Source: CAD feature listing. Evaluate the final solid. Frame: model axes, mm. Face numbers are marked on the shaded views. A direction names the side the tool comes from. Round coordinates to 2 decimals unless told otherwise and drop trailing zeros. Loops run counter-clockwise (first coordinate to the right, second up) from the corner with the lowest first, then second, coordinate; pieces in that order, holes last.
(1) First-contact query: pin 1 Ø8.5 at (x, z) = (-58.5, 8.5) entering from +Y; pin 2 Ø6 at (y, z) = (6.5, 10) entering from -X; pin 3 Ø2 at (x, z) = (-2, 17) entering from -Y; pin 4 Ø5 at (x, z) = (78.5, 0) entering from +Y. Flat tips, straight axial feed; report the tip coordinate or a pass-through.
(2) Section D-D, the plane x = -78.5. Return the cut outline in (y, z).
(3) Section A-A, the plane y = 2.5. Count the separate pieces of the cut face and the enclosed holes in it, plus the area to 3 significant figures.
(4) Section B-B, the plane x = 5. Return the cut outline in (y, z), plus the area to 3 significant figures.
(5) Set-up query: the marked faces 1, 2, 3, 4 and 5. Return all of +Z, -Z, +X, -X, +Y, -Y with unobstructed straight access to the full face (end or side cutting, diameter ignored); none if empty.
(6) Material intervals for probe 1 along Z at (x, y) = (58.5, 1.6); probe 2 along X at (y, z) = (1.15, 8.5); probe 3 along X at (y, z) = (6.25, -3), sorted ascending.
(7) Mould query, pull axis X, two halves, no side actions, for the marked faces 6, 7, 8 and 9. Classes: pulls with the +X half, pulls with the -X half, needs draft (parallel to the pull), parting line crosses it, or undercut.
(8) Section C-C, the plane x = 58.5. Return the cut outline in (y, z), plus the area to 3 significant figures.
```python
from build123d import *

# Parameters (mm, degrees)
SKETCH1_R                      = 1.8
BOSS_EXTRUDE1_DEPTH            = 6
BOSS_EXTRUDE2_DEPTH            = 40
CUT_EXTRUDE1_REACH             = 93.281
SKETCH3_W                      = 20
SKETCH3_H                      = 12.5
SKETCH4_R                      = 3.25
CUT_EXTRUDE2_DEPTH             = 12
CUT_EXTRUDE3_REACH             = 100.429
CUT_EXTRUDE4_START             = -2
SKETCH6_W                      = 35
SKETCH6_H                      = 27
CUT_EXTRUDE4_DEPTH             = 4.307692
FILLET1_R                      = 2
BOSS_EXTRUDE3_DEPTH            = 4
CUT_EXTRUDE5_REACH             = 93.658
CUT_EXTRUDE5_DIRECTION_2_REACH = 93.658
SKETCH10_W                     = 29
SKETCH10_H                     = 27
CUT_EXTRUDE7_DEPTH             = 1


with BuildPart() as part:
    # Sketch1 → Boss-Extrude1 (new body)
    with BuildSketch(Plane(origin=(0, 0, 0), x_dir=(1, 0, 0), z_dir=(0, 1, 0))):
        Polygon((68.5, 20), (68.5, 7.5), (88.5, 7.5), (88.5, -7.5), (68.5, -7.5), (68.5, -20), (-68.5, -20), (-68.5, -7.5), (-88.5, -7.5), (-88.5, 7.5), (-68.5, 7.5), (-68.5, 20), align=None)
        with Locations(Location((-78.5, 0, 0), (0, 0, 270))):
            Circle(SKETCH1_R, mode=Mode.SUBTRACT)
        with Locations(Location((-58.5, 8.5, 0), (0, 0, 270))):
            Circle(SKETCH1_R, mode=Mode.SUBTRACT)
        with Locations(Location((-58.5, -8.5, 0), (0, 0, 270))):
            Circle(SKETCH1_R, mode=Mode.SUBTRACT)
        with Locations(Location((58.5, -8.5, 0), (0, 0, 90))):
            Circle(SKETCH1_R, mode=Mode.SUBTRACT)
        with Locations(Location((78.5, 0, 0), (0, 0, 90))):
            Circle(SKETCH1_R, mode=Mode.SUBTRACT)
        with Locations(Location((58.5, 8.5, 0), (0, 0, 90))):
            Circle(SKETCH1_R, mode=Mode.SUBTRACT)
    extrude(amount=BOSS_EXTRUDE1_DEPTH)

    # Sketch2 → Boss-Extrude2 (add)
    with BuildSketch(Plane(origin=(0, 0, -20), x_dir=(-1, 0, 0), z_dir=(0, 0, -1))):
        Polygon((-88.5, 6), (88.5, 6), (88.5, 9), (35, 12), (25, 16), (-25, 16), (-35, 12), (-88.5, 9), align=None)
    extrude(amount=-BOSS_EXTRUDE2_DEPTH)

    # Sketch3 → Cut-Extrude1 (cut, up to next)
    with BuildSketch(Plane.XZ.offset(-6), mode=Mode.PRIVATE) as cut_extrude1_sk1:
        with Locations((-78.5, 13.75)):
            Rectangle(SKETCH3_W, SKETCH3_H)
    cut_extrude1_tool1 = extrude(cut_extrude1_sk1.sketch, amount=-CUT_EXTRUDE1_REACH, mode=Mode.PRIVATE) & part.part
    # Sketch3 → Cut-Extrude1 (cut, up to next)
    with BuildSketch(Plane.XZ.offset(-6), mode=Mode.PRIVATE) as cut_extrude1_sk2:
        with Locations((-78.5, -13.75)):
            Rectangle(SKETCH3_W, SKETCH3_H)
    cut_extrude1_tool2 = extrude(cut_extrude1_sk2.sketch, amount=-CUT_EXTRUDE1_REACH, mode=Mode.PRIVATE) & part.part
    # Sketch3 → Cut-Extrude1 (cut, up to next)
    with BuildSketch(Plane.XZ.offset(-6), mode=Mode.PRIVATE) as cut_extrude1_sk3:
        with Locations((78.5, 13.75)):
            Rectangle(SKETCH3_W, SKETCH3_H)
    cut_extrude1_tool3 = extrude(cut_extrude1_sk3.sketch, amount=-CUT_EXTRUDE1_REACH, mode=Mode.PRIVATE) & part.part
    # Sketch3 → Cut-Extrude1 (cut, up to next)
    with BuildSketch(Plane.XZ.offset(-6), mode=Mode.PRIVATE) as cut_extrude1_sk4:
        with Locations((78.5, -13.75)):
            Rectangle(SKETCH3_W, SKETCH3_H)
    cut_extrude1_tool4 = extrude(cut_extrude1_sk4.sketch, amount=-CUT_EXTRUDE1_REACH, mode=Mode.PRIVATE) & part.part
    add(cut_extrude1_tool1.solids().sort_by_distance((-78.5, 6, 13.75))[0], mode=Mode.SUBTRACT)
    add(cut_extrude1_tool2.solids().sort_by_distance((-78.5, 6, -13.75))[0], mode=Mode.SUBTRACT)
    add(cut_extrude1_tool3.solids().sort_by_distance((78.5, 6, 13.75))[0], mode=Mode.SUBTRACT)
    add(cut_extrude1_tool4.solids().sort_by_distance((78.5, 6, -13.75))[0], mode=Mode.SUBTRACT)

    # Sketch4 → Cut-Extrude2 (cut)
    with BuildSketch(Plane(origin=(0, 16, 0), x_dir=(1, 0, 0), z_dir=(0, 1, 0))):
        with Locations(Location((-58.5, 8.5, 0), (0, 0, 180))):
            Circle(SKETCH4_R)
        with Locations(Location((-78.5, 0, 0), (0, 0, 180))):
            Circle(SKETCH4_R)
        with Locations(Location((-58.5, -8.5, 0), (0, 0, 180))):
            Circle(SKETCH4_R)
        with Locations(Location((58.5, 8.5, 0), (0, 0, 180))):
            Circle(SKETCH4_R)
        with Locations(Location((58.5, -8.5, 0), (0, 0, 180))):
            Circle(SKETCH4_R)
        with Locations(Location((78.5, 0, 0), (0, 0, 180))):
            Circle(SKETCH4_R)
    extrude(amount=-CUT_EXTRUDE2_DEPTH, mode=Mode.SUBTRACT)

    # Sketch5 → Cut-Extrude3 (cut, up to next)
    with BuildSketch(Plane(origin=(0, 0, -20), x_dir=(-1, 0, 0), z_dir=(0, 0, -1)), mode=Mode.PRIVATE) as cut_extrude3_sk1:
        Polygon((-22.5, 0), (-16, 10), (16, 10), (22.5, 0), align=None)
    cut_extrude3_tool1 = extrude(cut_extrude3_sk1.sketch, amount=-CUT_EXTRUDE3_REACH, mode=Mode.PRIVATE) & part.part
    add(cut_extrude3_tool1.solids().sort_by_distance((0, 4.718615, -20))[0], mode=Mode.SUBTRACT)

    # Sketch6 → Cut-Extrude4 (cut)
    with BuildSketch(Plane.XZ.offset(-10).offset(CUT_EXTRUDE4_START)):
        Rectangle(SKETCH6_W, SKETCH6_H)
    extrude(amount=CUT_EXTRUDE4_DEPTH, mode=Mode.SUBTRACT)

    # Fillet1
    fillet1_edges = [part.edges().sort_by_distance(p)[0] for p in [
        (-17.5, 12, 0),
        (17.5, 12, 0),
    ]]
    fillet(fillet1_edges, radius=FILLET1_R)

    # Sketch7 → Boss-Extrude3 (add)
    with BuildSketch(Plane(origin=(0, 0, -20), x_dir=(-1, 0, 0), z_dir=(0, 0, -1))):
        Polygon((-22.5, 0), (-15.75, -1), (-13.25, -1), (-13.25, 10), (-16, 10), align=None)
        Polygon((16, 10), (22.5, 0), (15.75, -1), (13.25, -1), (13.25, 10), align=None)
    boss_extrude3 = extrude(amount=-BOSS_EXTRUDE3_DEPTH)

    # Mirror1: Boss-Extrude3 across plane
    add(boss_extrude3.mirror(Plane.XY))

    # Sketch8 → Cut-Extrude5 (cut, up to next)
    with BuildSketch(Plane.XZ.offset(-12), mode=Mode.PRIVATE) as cut_extrude5_sk1:
        with BuildLine():
            Line((-12.5, 11.5), (-12.5, -11.5))
            ThreePointArc((-12.5, -11.5), (-14.5, -13.5), (-16.5, -11.5))
            Line((-16.5, -11.5), (-16.5, 11.5))
            ThreePointArc((-16.5, 11.5), (-14.5, 13.5), (-12.5, 11.5))
        make_face()
    cut_extrude5_tool1 = extrude(cut_extrude5_sk1.sketch, amount=-CUT_EXTRUDE5_REACH, mode=Mode.PRIVATE) & part.part
    # Sketch8 → Cut-Extrude5 (cut, up to next)
    with BuildSketch(Plane.XZ.offset(-12), mode=Mode.PRIVATE) as cut_extrude5_sk2:
        with BuildLine():
            Line((16.5, 11.5), (16.5, -11.5))
            ThreePointArc((16.5, -11.5), (14.5, -13.5), (12.5, -11.5))
            Line((12.5, -11.5), (12.5, 11.5))
            ThreePointArc((12.5, 11.5), (14.5, 13.5), (16.5, 11.5))
        make_face()
    cut_extrude5_tool2 = extrude(cut_extrude5_sk2.sketch, amount=-CUT_EXTRUDE5_REACH, mode=Mode.PRIVATE) & part.part
    add(cut_extrude5_tool1.solids().sort_by_distance((-14.5, 12, 0))[0], mode=Mode.SUBTRACT)
    add(cut_extrude5_tool2.solids().sort_by_distance((14.5, 12, 0))[0], mode=Mode.SUBTRACT)

    # Sketch8 → Cut-Extrude5 direction 2 (cut, up to next)
    with BuildSketch(Plane.XZ.offset(-12), mode=Mode.PRIVATE) as cut_extrude5_direction_2_sk1:
        with BuildLine():
            Line((-12.5, 11.5), (-12.5, -11.5))
            ThreePointArc((-12.5, -11.5), (-14.5, -13.5), (-16.5, -11.5))
            Line((-16.5, -11.5), (-16.5, 11.5))
            ThreePointArc((-16.5, 11.5), (-14.5, 13.5), (-12.5, 11.5))
        make_face()
    cut_extrude5_direction_2_tool1 = extrude(cut_extrude5_direction_2_sk1.sketch, amount=CUT_EXTRUDE5_DIRECTION_2_REACH, mode=Mode.PRIVATE) & part.part
    # Sketch8 → Cut-Extrude5 direction 2 (cut, up to next)
    with BuildSketch(Plane.XZ.offset(-12), mode=Mode.PRIVATE) as cut_extrude5_direction_2_sk2:
        with BuildLine():
            Line((16.5, 11.5), (16.5, -11.5))
            ThreePointArc((16.5, -11.5), (14.5, -13.5), (12.5, -11.5))
            Line((12.5, -11.5), (12.5, 11.5))
            ThreePointArc((12.5, 11.5), (14.5, 13.5), (16.5, 11.5))
        make_face()
    cut_extrude5_direction_2_tool2 = extrude(cut_extrude5_direction_2_sk2.sketch, amount=CUT_EXTRUDE5_DIRECTION_2_REACH, mode=Mode.PRIVATE) & part.part
    add(cut_extrude5_direction_2_tool1.solids().sort_by_distance((-14.5, 12, 0))[0], mode=Mode.SUBTRACT)
    add(cut_extrude5_direction_2_tool2.solids().sort_by_distance((14.5, 12, 0))[0], mode=Mode.SUBTRACT)

    # Sketch10 → Cut-Extrude7 (cut)
    with BuildSketch(Plane(origin=(0, 16, 0), x_dir=(1, 0, 0), z_dir=(0, 1, 0))):
        Rectangle(SKETCH10_W, SKETCH10_H)
    extrude(amount=-CUT_EXTRUDE7_DEPTH, mode=Mode.SUBTRACT)


solid = part.part
```
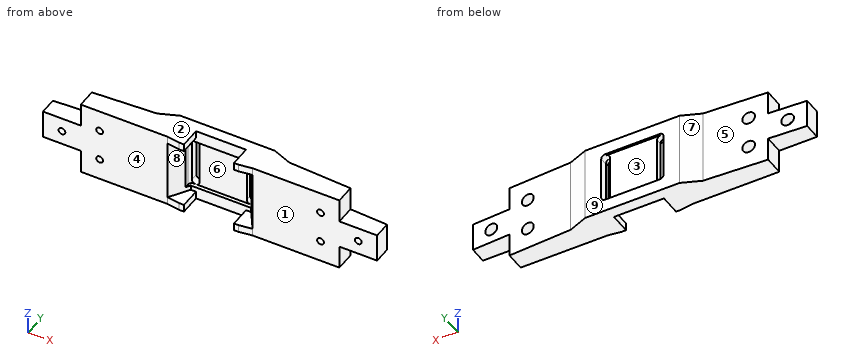
Output values:
1. pin 1: stops at y = 10.92
1. pin 2: stops at x = -88.5
1. pin 3: stops at y = 10
1. pin 4: stops at y = 4
2. outline: (0, -7.5) - (9.56, -7.5) - (9.56, -3.25) - (4, -3.25) - (4, -1.8) - (0, -1.8) - close; (0, 1.8) - (4, 1.8) - (4, 3.25) - (9.56, 3.25) - (9.56, 7.5) - (0, 7.5) - close
3. separate pieces: 2
3. enclosed holes: 6
3. area: 4,470 mm2
4. outline: (10, -20) - (16, -20) - (16, -13.5) - (15, -13.5) - (15, 13.5) - (16, 13.5) - (16, 20) - (10, 20) - (10, 13.5) - (12, 13.5) - (12, -13.5) - (10, -13.5) - close
4. area: 159 mm2
5. face 1: +Z, -Z, +X, -Y
5. face 2: +Z, +X, -X, +Y, -Y
5. face 3: +Y
5. face 4: +Z, -Z, -X, -Y
5. face 5: +Z, -Z, -X, +Y
6. probe 1: z = -20 to -10.3, -6.7 to 6.7, 10.3 to 20
6. probe 2: x = -68.5 to -60.3, -56.7 to -21.75, 21.75 to 56.7, 60.3 to 68.5
6. probe 3: x = -88.5 to -79.75, -77.25 to -18.44, 18.44 to 77.25, 79.75 to 88.5
7. face 6: undercut
7. face 7: pulls with the -X half
7. face 8: undercut
7. face 9: needs draft
8. outline: (0, -20) - (10.68, -20) - (10.68, -11.75) - (4, -11.75) - (4, -10.3) - (0, -10.3) - close; (0, -6.7) - (4, -6.7) - (4, -5.25) - (10.68, -5.25) - (10.68, 5.25) - (4, 5.25) - (4, 6.7) - (0, 6.7) - close; (0, 10.3) - (4, 10.3) - (4, 11.75) - (10.68, 11.75) - (10.68, 20) - (0, 20) - close
8. area: 312 mm2
